```python
from build123d import *

# Parameters (mm, degrees)
F0_R     = 1.9
F0_R_2   = 1
F1_DEPTH = 6
F2_R     = 0.4


with BuildPart() as f1:
    # F0 (on Top) → F1 (new body)
    with BuildSketch(Plane.XY):
        Circle(F0_R)
        Circle(F0_R_2, mode=Mode.SUBTRACT)
    extrude(amount=F1_DEPTH)

    # F2
    f2_edges = [f1.edges().sort_by_distance(p)[0] for p in [
        (-1.9, 0, 6),
    ]]
    fillet(f2_edges, radius=F2_R)

    # F3 (on Front) → F4 (revolve)
    with BuildSketch(Plane.XZ):
        with BuildLine():
            Line((-1.9, 3.85359), (-1.9, 4.8))
            Line((-1.9, 4.8), (-2.273205, 4.15359))
            ThreePointArc((-2.273205, 4.15359), (-2.273205, 3.95359), (-2.1, 3.85359))
            Line((-2.1, 3.85359), (-1.9, 3.85359))
        make_face()
        with BuildLine():
            Line((-2.1, 2.45359), (-1.9, 2.45359))
            Line((-1.9, 2.45359), (-1.9, 3.4))
            Line((-1.9, 3.4), (-2.273205, 2.75359))
            ThreePointArc((-2.273205, 2.75359), (-2.273205, 2.55359), (-2.1, 2.45359))
        make_face()
        with BuildLine():
            Line((-2.1, 1.05359), (-1.9, 1.05359))
            Line((-1.9, 1.05359), (-1.9, 2))
            Line((-1.9, 2), (-2.273205, 1.35359))
            ThreePointArc((-2.273205, 1.35359), (-2.273205, 1.15359), (-2.1, 1.05359))
        make_face()
    revolve(axis=Axis((0, 0, 2.84007), (0, 0, -1)))


solid = f1.part
```
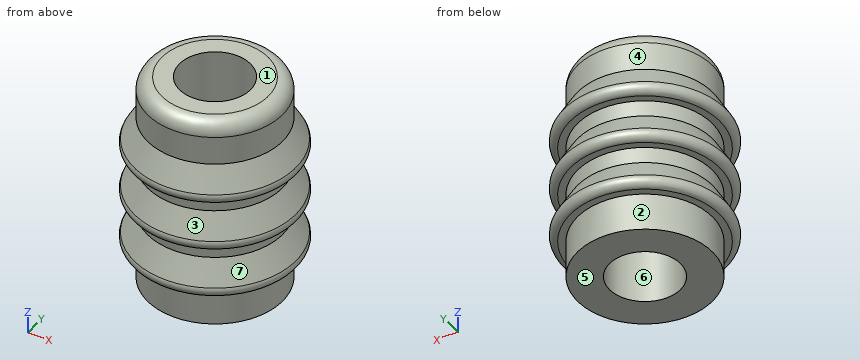
For this review, take the finished solid that the model builds, in its own axes (mm). Face numbers are marked on the shaded views. A direction names the side the tool comes from. Coordinates: 2 decimals unless noted, no trailing zeros. Loops run counter-clockwise (first coordinate to the right, second up) from the corner with the lowest first, then second, coordinate; pieces in that order, holes last. Notation, with made-up numbers: (27, 21.5) -> (62, 21.5) arc R29 ccw to (62, 50.5) -> close; hole circle Ø6 at (28, 28). An arc over 180 degrees is marked (long way). Return JSON: item names as keys, results as strings. Group by question number.
(1) Tool access review of the marked faces 1, 2, 3 and 4: name each direction out of +Z, -Z, +X, -X, +Y, -Y from which nothing blocks a thin tool from reaching the whole face with its end or side.
(2) Consider section D-D, the plane z = 2.55. Give the boundary of the cut face in (x, y), plus the area to 3 significant figures.
(3) Mouldability with a two-part tool opening along Z and no side actions: class the marked faces 5, 6 and 7 as pulls with the +Z half, pulls with the -Z half, needs draft (parallel to the pull), parting line crosses it, or undercut.
(4) To check wall thickness, follow L1, parallel to Z at x = 1.9, y = -0.55; L2, parallel to Z at x = 1.25, y = 1.55; L3, parallel to Y at x = 0, z = 3.7. State the ranges of each line that lie inside material, in increasing order.
(5) Consider section C-C, the plane z = 0.8. Give the boundary of the cut face in (x, y), plus the area to 3 significant figures.
Results below:
{
 "1": {"face 1": "+Z, +X, -X, +Y, -Y", "face 2": "-Z", "face 3": "none", "face 4": "+Z"},
 "2": {"outline": "circle Ø4.54 at (0, 0); hole circle Ø2 at (0, 0)", "area": "13.1 mm2"},
 "3": {"face 5": "pulls with the -Z half", "face 6": "needs draft", "face 7": "undercut"},
 "4": {"L1": "z = 1.05 to 1.86, 2.45 to 3.26, 3.85 to 4.66", "L2": "z = 1.05 to 1.84, 2.45 to 3.24, 3.85 to 4.64", "L3": "y = -1.9 to -1, 1 to 1.9"},
 "5": {"outline": "circle Ø3.8 at (0, 0); hole circle Ø2 at (0, 0)", "area": "8.20 mm2"}
}
